Autodesk Inventor part; units mm, degrees
ref_plane "YZ Plane" through (0, 0, 0) normal (1, 0, 0) x (0, 1, 0)
ref_plane "XZ Plane" through (0, 0, 0) normal (0, 1, 0) x (-1, 0, 0)
ref_plane "XY Plane" through (0, 0, 0) normal (0, 0, 1) x (1, 0, 0)
sketch "Sketch1" plane through (0, 0, 0) normal (0, 0, 1) x (1, 0, 0)
  circle A0 centre (0, 0) radius 47.625
  dimension "d0" = 95.25
extrude "Extrusion1" add sketch "Sketch1" along normal blind 6.35
sketch "Sketch2" plane through (0, 0, 6.35) normal (0, 0, 1) x (1, 0, 0)
  circle A0 centre (0, 0) radius 25.4
  dimension "d3" = 50.8
extrude "Extrusion2" cut sketch "Sketch2" against normal blind 6.35
sketch "Sketch3" plane through (0, 0, 6.35) normal (0, 0, 1) x (1, 0, 0)
  line L0 (0, 0) -> (-44.45, 0)
  circle A0 centre (-44.45, 0) radius 1.905
  circle A1 centre (-22.225, -38.4948) radius 1.905
  circle A2 centre (22.225, -38.4948) radius 1.905
  circle A3 centre (44.45, 0) radius 1.905
  circle A4 centre (22.225, 38.4948) radius 1.905
  circle A5 centre (-22.225, 38.4948) radius 1.905
  dimension "d6" = 3.81
  dimension "d7" = 44.45
  dimension "d10" = 360
extrude "Extrusion3" cut sketch "Sketch3" against normal blind 6.35
chamfer "Chamfer1" distance 1.27 angle 45 6 edges at (-24.13, 38.4948, 6.35) (-46.355, 0, 6.35) (-24.13, -38.4948, 6.35) (20.32, 38.4948, 6.35) (42.545, 0, 6.35) (20.32, -38.4948, 6.35)
sketch "Sketch4" plane through (0, 0, 6.35) normal (0, 0, 1) x (1, 0, 0)
  circle A0 centre (0, 41.91) radius 1.8415
  circle A1 centre (-36.2951, 20.955) radius 1.8415
  circle A2 centre (-36.2951, -20.955) radius 1.8415
  circle A3 centre (0, -41.91) radius 1.8415
  circle A4 centre (36.2951, -20.955) radius 1.8415
  circle A5 centre (36.2951, 20.955) radius 1.8415
  point P0 (0, 0)
  dimension "d17" = 3.683
  dimension "d18" = 41.91
  dimension "d21" = 360
extrude "Extrusion4" cut sketch "Sketch4" against normal blind 25.4
sketch "Sketch5" plane through (0, 0, 0) normal (0, 0, -1) x (-1, 0, 0)
  circle A0 centre (0, 41.91) radius 1.8415
  line L0 (-3.8861, 41.91) -> (-1.9431, 45.2755)
  line L1 (-1.9431, 45.2755) -> (1.9431, 45.2755)
  line L2 (1.9431, 45.2755) -> (3.8861, 41.91)
  line L3 (3.8861, 41.91) -> (1.9431, 38.5445)
  line L4 (1.9431, 38.5445) -> (-1.9431, 38.5445)
  line L5 (-1.9431, 38.5445) -> (-3.8861, 41.91)
  line L6 (-38.2382, 17.5895) -> (-40.1813, 20.955)
  line L7 (-40.1813, 20.955) -> (-38.2382, 24.3205)
  line L8 (-38.2382, 24.3205) -> (-34.3521, 24.3205)
  line L9 (-34.3521, 24.3205) -> (-32.409, 20.955)
  line L10 (-32.409, 20.955) -> (-34.3521, 17.5895)
  line L11 (-34.3521, 17.5895) -> (-38.2382, 17.5895)
  line L12 (-34.3521, -24.3205) -> (-38.2382, -24.3205)
  line L13 (-38.2382, -24.3205) -> (-40.1813, -20.955)
  line L14 (-40.1813, -20.955) -> (-38.2382, -17.5895)
  line L15 (-38.2382, -17.5895) -> (-34.3521, -17.5895)
  line L16 (-34.3521, -17.5895) -> (-32.409, -20.955)
  line L17 (-32.409, -20.955) -> (-34.3521, -24.3205)
  line L18 (3.8861, -41.91) -> (1.9431, -45.2755)
  line L19 (1.9431, -45.2755) -> (-1.9431, -45.2755)
  line L20 (-1.9431, -45.2755) -> (-3.8861, -41.91)
  line L21 (-3.8861, -41.91) -> (-1.9431, -38.5445)
  line L22 (-1.9431, -38.5445) -> (1.9431, -38.5445)
  line L23 (1.9431, -38.5445) -> (3.8861, -41.91)
  line L24 (38.2382, -17.5895) -> (40.1813, -20.955)
  line L25 (40.1813, -20.955) -> (38.2382, -24.3205)
  line L26 (38.2382, -24.3205) -> (34.3521, -24.3205)
  line L27 (34.3521, -24.3205) -> (32.409, -20.955)
  line L28 (32.409, -20.955) -> (34.3521, -17.5895)
  line L29 (34.3521, -17.5895) -> (38.2382, -17.5895)
  line L30 (34.3521, 24.3205) -> (38.2382, 24.3205)
  line L31 (38.2382, 24.3205) -> (40.1813, 20.955)
  line L32 (40.1813, 20.955) -> (38.2382, 17.5895)
  line L33 (38.2382, 17.5895) -> (34.3521, 17.5895)
  line L34 (34.3521, 17.5895) -> (32.409, 20.955)
  line L35 (32.409, 20.955) -> (34.3521, 24.3205)
  point P0 (0, 0)
  point P1 (-36.2951, 20.955)
  point P2 (-36.2951, -20.955)
  point P3 (0, -41.91)
  point P4 (36.2951, -20.955)
  point P5 (36.2951, 20.955)
  dimension "d25" = 6.731
  dimension "d28" = 360
extrude "Extrusion5" cut sketch "Sketch5" against normal blind 2.3813
sketch "Sketch6" plane through (0, 0, 6.35) normal (0, 0, 1) x (1, 0, 0)
  circle A0 centre (20.795, 25.8191) radius 3.175
  line L0 (0, 0) -> (0, 9.7848)
  circle A1 centre (-20.795, 25.8191) radius 3.175
  dimension "d32" = 6.35
  dimension "d33" = 20.795
  dimension "d34" = 25.8191
extrude "Extrusion6" cut sketch "Sketch6" against normal blind 25.4
sketch "Sketch7" plane through (0, 0, 0) normal (0, 0, -1) x (-1, 0, 0)
  circle A0 centre (-20.795, 25.8191) radius 3.175
  circle A1 centre (20.795, 25.8191) radius 3.175
  line L0 (32.409, 20.955) -> (34.3521, 24.3205)
  line L1 (34.3521, 24.3205) -> (38.2382, 24.3205)
  line L2 (38.2382, 24.3205) -> (40.1813, 20.955)
  line L3 (40.1813, 20.955) -> (38.2382, 17.5895)
  line L4 (38.2382, 17.5895) -> (34.3521, 17.5895)
  line L5 (34.3521, 17.5895) -> (32.409, 20.955)
  line L6 (1.9431, -38.5445) -> (3.8861, -41.91)
  line L7 (3.8861, -41.91) -> (1.9431, -45.2755)
  line L8 (1.9431, -45.2755) -> (-1.9431, -45.2755)
  line L9 (-1.9431, -45.2755) -> (-3.8861, -41.91)
  line L10 (-3.8861, -41.91) -> (-1.9431, -38.5445)
  line L11 (-1.9431, -38.5445) -> (1.9431, -38.5445)
  line L12 (-34.3521, 17.5895) -> (-38.2382, 17.5895)
  line L13 (-38.2382, 17.5895) -> (-40.1813, 20.955)
  line L14 (-40.1813, 20.955) -> (-38.2382, 24.3205)
  line L15 (-38.2382, 24.3205) -> (-34.3521, 24.3205)
  line L16 (-34.3521, 24.3205) -> (-32.409, 20.955)
  line L17 (-32.409, 20.955) -> (-34.3521, 17.5895)
  line L18 (-1.9431, 38.5445) -> (-3.8861, 41.91)
  line L19 (-3.8861, 41.91) -> (-1.9431, 45.2755)
  line L20 (-1.9431, 45.2755) -> (1.9431, 45.2755)
  line L21 (1.9431, 45.2755) -> (3.8861, 41.91)
  line L22 (3.8861, 41.91) -> (1.9431, 38.5445)
  line L23 (1.9431, 38.5445) -> (-1.9431, 38.5445)
  line L24 (-32.409, -20.955) -> (-34.3521, -24.3205)
  line L25 (-34.3521, -24.3205) -> (-38.2382, -24.3205)
  line L26 (-38.2382, -24.3205) -> (-40.1813, -20.955)
  line L27 (-40.1813, -20.955) -> (-38.2382, -17.5895)
  line L28 (-38.2382, -17.5895) -> (-34.3521, -17.5895)
  line L29 (-34.3521, -17.5895) -> (-32.409, -20.955)
  line L30 (34.3521, -17.5895) -> (38.2382, -17.5895)
  line L31 (38.2382, -17.5895) -> (40.1813, -20.955)
  line L32 (40.1813, -20.955) -> (38.2382, -24.3205)
  line L33 (38.2382, -24.3205) -> (34.3521, -24.3205)
  line L34 (34.3521, -24.3205) -> (32.409, -20.955)
  line L35 (32.409, -20.955) -> (34.3521, -17.5895)
  circle A2 centre (-22.225, 38.4948) radius 1.905
  circle A3 centre (-22.225, -38.4948) radius 1.905
  circle A4 centre (44.45, 0) radius 1.905
  circle A5 centre (22.225, -38.4948) radius 1.905
  circle A6 centre (-44.45, 0) radius 1.905
  circle A7 centre (22.225, 38.4948) radius 1.905
  circle A8 centre (0, 0) radius 25.4
  circle A9 centre (0, 0) radius 47.625
  circle A10 centre (0, 0) radius 36.327
extrude "Extrusion7" cut sketch "Sketch7" against normal blind 25.4 contours A10
sketch "Sketch8" plane through (0, 0, 6.35) normal (0, 0, 1) x (1, 0, 0)
  circle A0 centre (0, 0) radius 47.117
  circle A1 centre (0, 0) radius 47.625
  dimension "d39" = 94.234
  dimension "d40" = 95.25
extrude "PRINT_FEATURE1" [suppressed]
properties part number "aftSectionAirtightCap" material "ABS Plastic"
Geometry check sheet. Reference: the model listing, model coordinates, mm. A direction names the side the tool comes from. Round coordinates to 2 decimals unless told otherwise and drop trailing zeros. Loops run counter-clockwise (first coordinate to the right, second up) from the corner with the lowest first, then second, coordinate; pieces in that order, holes last.
Item 1: Cross-section at A-A on y = 0. Count the separate pieces of the cut face and the enclosed holes in it, then the cut area to 3 significant figures.
Item 2: Mould release check, pull along Y, two halves, no side actions. Record for faces 1 (the cylindrical face through (-37.794, 28.979, 3.131)), 2 (the cylindrical face through (-42.633, 0.572, 2.576)): pulls with the +Y half, pulls with the -Y half, needs draft (parallel to the pull), parting line crosses it, or undercut.
Item 3: Cross-section at D-D on y = -14.5. Record the boundary of the cut face in (x, z), then the cut area to 3 significant figures.
Item 4: Thickness scan on line 1 (Y direction, x = 1.5, z = 5.25); line 2 (X direction, y = -1, z = 1.5); line 3 (X direction, y = 38.5, z = 2.5). Record the ranges inside material, lowest first.
Item 5: Access from +Z, -Z, +X, -X, +Y, -Y to the whole of each face (thin tool, end or side, straight path). Record for faces 3 (the flat face through (33.394, 22.661, 1.174)), 4 (the cylindrical face through (-0.399, 40.112, 4.393)).
Item 6: Cross-section at B-B on x = -30.5. Record the boundary of the cut face in (y, z), then the cut area to 3 significant figures.
Item 7: Gauge pin test, flat ends, axial feed: pin 1 (3 mm diameter, centred on x = -36.3, y = 20.96, fed in from -Z); pin 2 (2 mm diameter, centred on x = 35.5, y = -19.5, fed in from -Z); pin 3 (2 mm diameter, centred on x = 4, z = 2.5, fed in from +Y); pin 4 (1.2 mm diameter, centred on x = -36.5, z = 1.5, fed in from +Y). Record the tip position at first contact, or that the pin passes through.
Answer sheet:
1. separate pieces: 4
1. enclosed holes: 0
1. area: 91.9 mm2
2. face 1: parting line crosses it
2. face 2: undercut
3. outline: (-45.36, 0) - (-33.31, 0) - (-33.31, 6.35) - (-45.36, 6.35) - close; (33.31, 0) - (45.36, 0) - (45.36, 6.35) - (33.31, 6.35) - close
3. area: 153 mm2
4. line 1: y = -47.6 to -42.98, -40.84 to -36.3, 36.3 to 40.84, 42.98 to 47.6
4. line 2: x = -47.61 to -46.07, -42.83 to -36.31, 36.31 to 42.83, 46.07 to 47.61
4. line 3: x = -28.03 to -24.13, -20.32 to 20.32, 24.13 to 28.03
5. face 3: -Z
5. face 4: +Z, -Z
6. outline: (-36.58, 0) - (-19.73, 0) - (-19.73, 6.35) - (-36.58, 6.35) - close; (19.73, 0) - (36.58, 0) - (36.58, 6.35) - (19.73, 6.35) - close
6. area: 214 mm2
7. pin 1: passes through
7. pin 2: stops at z = 2.38
7. pin 3: stops at y = 47.53
7. pin 4: stops at y = 31.29
